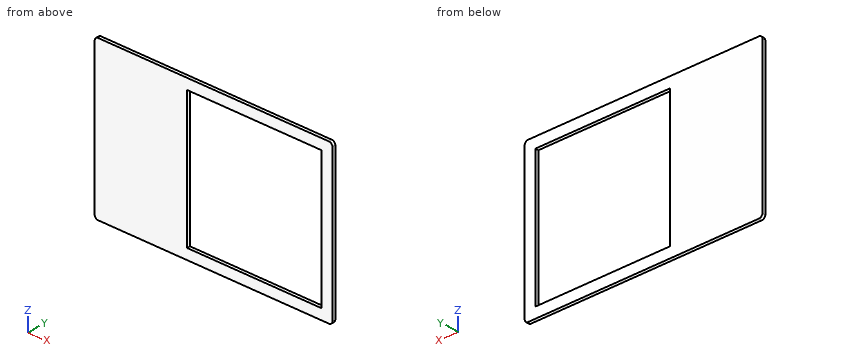
from build123d import *

# Parameters (mm, degrees)
F1_DEPTH = 2.5
F2_DEPTH = 2.5
F3_DEPTH = 2.5
F0_W     = 102.1108726621
F0_H     = 8
F4_DEPTH = 2.5
F5_DEPTH = 2.5
F6_R     = 2.5
F7_R     = 2.5
F8_R     = 2.5
F9_R     = 2.5


with BuildPart() as f1:
    # F0 (on Front) → F1 (new body)
    with BuildSketch(Plane.XZ):
        Polygon((-20.1, 60), (-90.1, 60), (-90.1, -60), (-20.1, -60), (-20.1, -52), (-20.1, 52), align=None)
    extrude(amount=F1_DEPTH)

    # F0 (on Front) → F2 (join)
    with BuildSketch(Plane.XZ):
        Polygon((90.1, 60), (-20.1, 60), (-20.1, 52), (82.0108726621, 52), (90.1, 52), align=None)
    extrude(amount=F2_DEPTH)

    # F0 (on Front) → F3 (join)
    with BuildSketch(Plane.XZ):
        Polygon((90.1, -60), (90.1, 52), (82.0108726621, 52), (82.0108726621, -52), (82.0108726621, -60), align=None)
    extrude(amount=F3_DEPTH)

    # F0 (on Front) → F4 (join)
    with BuildSketch(Plane.XZ):
        with Locations((30.955436331, -56)):
            Rectangle(F0_W, F0_H)
    extrude(amount=F4_DEPTH)

    # F0 (on Front) → F5 (join)
    with BuildSketch(Plane.XZ):
        Polygon((90.1, -60), (90.1, 52), (82.0108726621, 52), (82.0108726621, -52), (82.0108726621, -60), align=None)
    extrude(amount=F5_DEPTH)

    # F6
    f6_edges = [f1.edges().sort_by_distance(p)[0] for p in [
        (-90.1, -1.25, 60),
    ]]
    fillet(f6_edges, radius=F6_R)

    # F7
    f7_edges = [f1.edges().sort_by_distance(p)[0] for p in [
        (90.1, -1.25, 60),
    ]]
    fillet(f7_edges, radius=F7_R)

    # F8
    f8_edges = [f1.edges().sort_by_distance(p)[0] for p in [
        (90.1, -1.25, -60),
    ]]
    fillet(f8_edges, radius=F8_R)

    # F9
    f9_edges = [f1.edges().sort_by_distance(p)[0] for p in [
        (-90.1, -1.25, -60),
    ]]
    fillet(f9_edges, radius=F9_R)


solid = f1.part
For this review, take the finished solid that the model builds, in its own axes (mm). Coordinates: 2 decimals unless noted, no trailing zeros. Loops run counter-clockwise (first coordinate to the right, second up) from the corner with the lowest first, then second, coordinate; pieces in that order, holes last. Notation, with made-up numbers: (-2.75, 83.5) - (14.25, 83.5) arc R10 ccw to (14.25, 92.5) - close; hole circle Ø11 at (-30.75, 0.25). An arc over 180 degrees is marked (long way). Use a Markdown table: item, result. Add a question column.
Item 1: We need section A-A (z = 6.5). Give the boundary of the cut face in (x, y).
Item 2: We need section B-B (x = 59.5). Give the boundary of the cut face in (y, z).
Item 3: For line 1 (X direction, y = -0.7, z = 34.5); line 2 (Z direction, x = 30, y = -2.1), list the stretches that pass through material, from the lowest coordinate up.
Item 4: We need section C-C (y = -1.7). Give the boundary of the cut face in (x, z).
Results list:
| question | item | result |
|---|---|---|
| 1 | outline | (-90.1, -2.5) - (-20.1, -2.5) - (-20.1, 0) - (-90.1, 0) - close; (82.01, -2.5) - (90.1, -2.5) - (90.1, 0) - (82.01, 0) - close |
| 2 | outline | (-2.5, -60) - (0, -60) - (0, -52) - (-2.5, -52) - close; (-2.5, 52) - (0, 52) - (0, 60) - (-2.5, 60) - close |
| 3 | line 1 | x = -90.1 to -20.1, 82.01 to 90.1 |
| 3 | line 2 | z = -60 to -52, 52 to 60 |
| 4 | outline | (-90.1, -57.5) arc R2.5 ccw to (-87.6, -60) - (87.6, -60) arc R2.5 ccw to (90.1, -57.5) - (90.1, 57.5) arc R2.5 ccw to (87.6, 60) - (-87.6, 60) arc R2.5 ccw to (-90.1, 57.5) - close; hole (-20.1, -52) - (82.01, -52) - (82.01, 52) - (-20.1, 52) - close |
